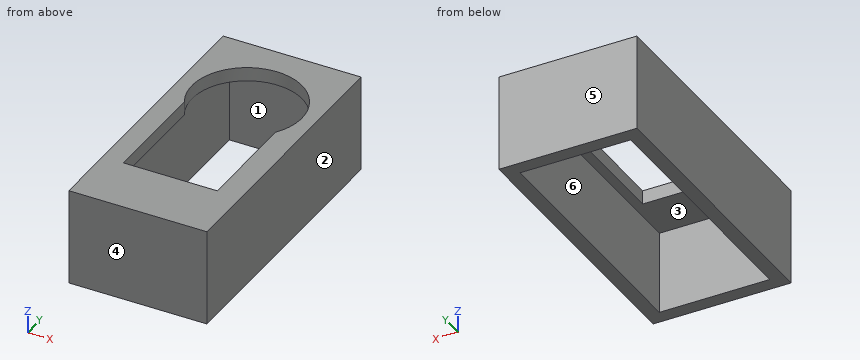
Autodesk Fusion 360 part; units mm, degrees
sketch "Sketch1" plane through (0, 0, 0) normal (0, 0, 1) x (1, 0, 0)
  line L0 (0, 0) -> (12, 0)
  line L1 (12, 0) -> (12, 33)
  line L2 (12, 33) -> (0, 33)
  line L3 (0, 33) -> (0, 0)
  line L4 (-2, 35) -> (14, 35)
  line L5 (14, 35) -> (14, -2)
  line L6 (14, -2) -> (-2, -2)
  line L7 (-2, -2) -> (-2, 35)
  dimension "d1" = 33
  dimension "d2" = 12
  dimension "d3" = 2
  dimension "d4" = 2
  dimension "d5" = 2
  dimension "d6" = 2
extrude "Extrude1" add sketch "Sketch1" along normal blind 20 makes body 1
extrude "Extrude2" add sketch "Sketch1" against normal blind 2 contours L0 L1 L2 L3 | L4 L5 L6 L7 bodies 1
sketch "Sketch2" plane through (0, 0, 20) normal (0, 0, 1) x (-1, 0, 0)
  line L0 (0, 0) -> (0, -33)
  line L1 (0, -33) -> (-12, -33)
  line L2 (-12, -33) -> (-12, 0)
  line L3 (-12, 0) -> (0, 0)
  line L4 (2, 2) -> (-14, 2)
  line L5 (-14, 2) -> (-14, -35)
  line L6 (-14, -35) -> (2, -35)
  line L7 (2, -35) -> (2, 2)
  line L8 (4, 4) -> (-16, 4)
  line L9 (-16, 4) -> (-16, -37)
  line L10 (-16, -37) -> (4, -37)
  line L11 (4, -37) -> (4, 4)
  dimension "d11" = 2
extrude "Extrude3" add sketch "Sketch2" against normal blind 12 separate body contours L8 L9 L10 L11 makes body 2
sketch "Sketch3" plane through (0, 0, 20) normal (0, 0, 1) x (-1, 0, 0)
  line L0 (2, 2) -> (2, -35)
  line L1 (2, -35) -> (-14, -35)
  line L2 (-14, -35) -> (-14, 2)
  line L3 (-14, 2) -> (2, 2)
  line L4 (4, -37) -> (4, 4)
  line L5 (4, 4) -> (-16, 4)
  line L6 (-16, 4) -> (-16, -37)
  line L7 (-16, -37) -> (4, -37)
extrude "Extrude5" add sketch "Sketch3" along normal blind 2 contours L0 L1 L2 L3 | L4 L5 L6 L7 bodies 2
sketch "Sketch4" plane through (0, 0, 22) normal (0, 0, 1) x (-1, 0, 0)
  line L0 (-16, -37) -> (4, -37)
  line L1 (4, -37) -> (4, 4)
  line L2 (4, 4) -> (-16, 4)
  line L3 (-16, 4) -> (-16, -37)
  circle A0 centre (-6, -25) radius 7.9669
  line L4 (-12.5894, -20.5221) -> (-12.5894, -5)
  line L5 (-12.5894, -5) -> (1, -5)
  line L6 (1, -5) -> (1, -21.1958)
  dimension "d20" = 15.9338
extrude "Extrude6" cut sketch "Sketch4" against normal blind 2 contours A0 | A0 L4 L5 L6 bodies 2
hidden bodies 1
Design review of the part built by this model. Coordinates are the model's own, in mm. Face numbers are marked on the shaded views. A direction names the side the tool comes from. Give positions to 0.01 mm unless a question says otherwise; leave off trailing zeros. Write each loop counter-clockwise with the first axis right and the second up, starting at its lowest first coordinate (ties: lowest second). Pieces come first, ordered by that corner, then holes. Notation, with made-up numbers: M 83.25,-24.5 L 90.25,-24.5 A21 cw 90.25,-6.5 Z; hole C 1.25,3 d3. An arc over 180 degrees is marked long. Return JSON: item names as keys, results as strings. Group by question number.
Item 1: Take a section at D-D (y = -1). Give the boundary of the cut face in (x, z), plus the area to 3 significant figures.
Item 2: Take a section at A-A (y = 20). Give the boundary of the cut face in (x, z).
Item 3: Take a section at B-B (x = 6). Give the boundary of the cut face in (y, z).
Item 4: Wall thickness on line 1 along X through (y, z) = (25, 21.5); line 2 along Y through (x, z) = (12.25, 12.25); line 3 along Y through (x, z) = (6, 20.45): over which ranges is each line inside the solid? List them lowest first.
Item 5: Tool access review of the marked faces 5 and 6: name each direction out of +Z, -Z, +X, -X, +Y, -Y from which nothing blocks a thin tool from reaching the whole face with its end or side.
Item 6: The part is to be moulded in two halves that separate along Y. For the marked faces 1, 2, 3 and 4, say which applies: pulls with the +Y half, pulls with the -Y half, needs draft (parallel to the pull), parting line crosses it, or undercut.
Item 7: Take a section at C-C (z = 10.25). Give the boundary of the cut face in (x, y).
Return value:
{
 "1": {"outline": "M -4,8 L -2,8 L -2,20 L 14,20 L 14,8 L 16,8 L 16,22 L -4,22 Z", "area": "88.0 mm2"},
 "2": {"outline": "M -4,8 L -2,8 L -2,20 L -1,20 L -1,22 L -4,22 Z; M 12.59,20 L 14,20 L 14,8 L 16,8 L 16,22 L 12.59,22 Z"},
 "3": {"outline": "M -4,8 L -2,8 L -2,20 L 5,20 L 5,22 L -4,22 Z; M 32.97,20 L 35,20 L 35,8 L 37,8 L 37,22 L 32.97,22 Z"},
 "4": {"line 1": "x = -4 to -1.97, 13.97 to 16", "line 2": "y = -4 to -2, 35 to 37", "line 3": "y = -4 to 5, 32.97 to 37"},
 "5": {"face 5": "+Z, -Z, +X, -X, +Y", "face 6": "-Z"},
 "6": {"face 1": "undercut", "face 2": "needs draft", "face 3": "undercut", "face 4": "pulls with the -Y half"},
 "7": {"outline": "M -4,-4 L 16,-4 L 16,37 L -4,37 Z; hole M -2,-2 L 14,-2 L 14,35 L -2,35 Z"}
}
